Could you check a few things on this drawing? It's one solid part, dimensions in mm from its lowest x, y, z. Coordinates: 2 decimals unless noted, no trailing zeros. Write each loop counter-clockwise with the first axis right and the second up, starting at its lowest first coordinate (ties: lowest second). Pieces come first, ordered by that corner, then holes. Notation, with made-up numbers: M 21.25,66 L 54.25,66 A25 ccw 54.25,104 Z; hole C 31,-12.5 d10. An arc over 180 degrees is marked long. Use a Markdown table: item, result.
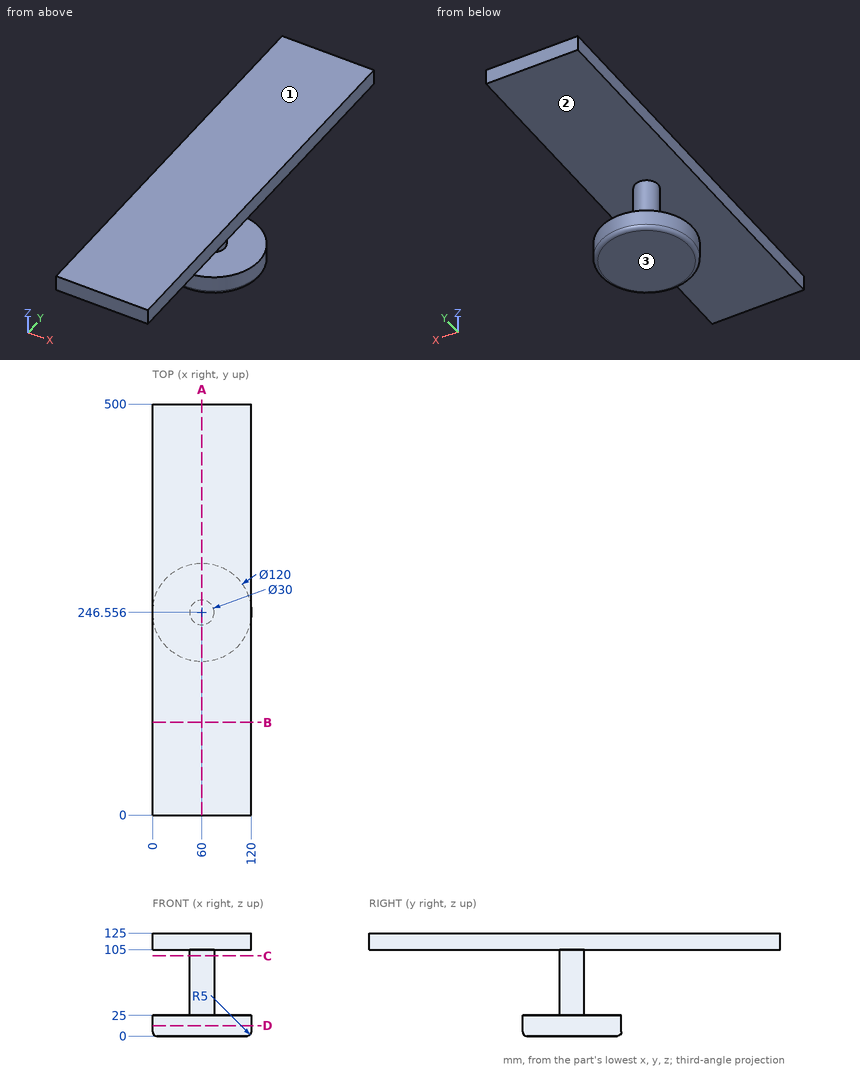
1. Suppose I cut it at C-C on z = 97.5. Write out the boundary of the cut face in (x, y) (1 decimal), and give its area (3 significant figures).
Answers follow:
| item | result |
|---|---|
| outline | C 60,246.6 d30 |
| area | 707 mm2 |
2. Suppose I cut it at A-A on x = 60. Write out the boundary of the cut face in (y, z) (1 decimal), and give its area (3 significant figures).
Answers follow:
| item | result |
|---|---|
| outline | M 0,105 L 231.6,105 L 231.6,25 L 186.6,25 L 186.6,5 A5 ccw 191.6,0 L 301.6,0 A5 ccw 306.6,5 L 306.6,25 L 261.6,25 L 261.6,105 L 500,105 L 500,125 L 0,125 Z |
| area | 15,400 mm2 |
3. Suppose I cut it at B-B on y = 113. Write out the boundary of the cut face in (x, z).
Answers follow:
| item | result |
|---|---|
| outline | M 0,105 L 120,105 L 120,125 L 0,125 Z |
4. I need wall thicknesses on probe 1 along Z at (x, y) = (47, 263.5); probe 2 along Y at (x, z) = (61, 69.5); probe 3 along Z at (x, y) = (43, 177). Which ranges of each line are inside material? Lowest first, please.
Answers follow:
| item | result |
|---|---|
| probe 1 | z = 0 to 25, 105 to 125 |
| probe 2 | y = 231.59 to 261.52 |
| probe 3 | z = 105 to 125 |
5. Suppose I cut it at D-D on z = 12.5. Write out the boundary of the cut face in (x, y) (1 decimal), and give its area (3 significant figures).
Answers follow:
| item | result |
|---|---|
| outline | C 60,246.6 d120 |
| area | 11,300 mm2 |
6. Will these pins go through, and if not, where does the flat tip stop? pin 1 Ø3 at (x, y) = (31, 57.5) entering from -Z; pin 2 Ø4 at (x, z) = (75, 76) entering from +Y; pin 3 Ø12 at (x, z) = (45.5, 23.5) entering from +Y.
Answers follow:
| item | result |
|---|---|
| pin 1 | stops at z = 105 |
| pin 2 | stops at y = 254.04 |
| pin 3 | stops at y = 305.95 |
7. We'd pull the mould along Z, two halves only. Please class the marked faces 1, 2 and 3: +Z half, -Z half, draft (parallel to the pull), parting line (faces both ways), or undercut.
Answers follow:
| item | result |
|---|---|
| face 1 | +Z half |
| face 2 | undercut |
| face 3 | -Z half |
